Can you work these out from the model? Positions are in its coordinate system, mm. A direction names the side the tool comes from. Round coordinates to 2 decimals unless told otherwise and drop trailing zeros. Write each loop counter-clockwise with the first axis right and the second up, starting at its lowest first coordinate (ties: lowest second). Pieces come first, ordered by that corner, then holes. Notation, with made-up numbers: (82, 64) - (110, 64) arc R21 ccw to (110, 76) - close; hole circle Ø11 at (48, -11.5). An arc over 180 degrees is marked (long way). One line per item, written item: value. Start each with the question number.
(1) I'm going to push flat-ended pins straight in: pin 1 Ø1.2 at (x, z) = (1, 66) entering from -Y; pin 2 Ø1 at (x, y) = (0.5, -17) entering from +Z; pin 3 Ø1.2 at (x, z) = (2, -78) entering from +Y. Where does each tip first touch, or does it pass through?
(2) I want a section at A-A on x = 3.05. List the corners of the cut face in (y, z) for me.
(3) If I drill on L1, parallel to Y at x = 2.6, z = -17.5; L2, parallel to Z at x = 1.5, y = -25; L3, parallel to Y at x = 3.15, z = 90, over which ranges is the centre line in solid material (lowest first)? Write a range as from..to.
(4) Thinking about a two-plate mould opening in Y: for faces 1 (the face through (4, 8, 1)), 2 (the face through (2, 23.8, -19.1)), 3 (the face through (2, -23.8, 19.1)), 4 (the face through (2.03, -14.51, -31.78)), which applies, +Y half, -Y half, draft (parallel to the pull), parting line (faces both ways), or undercut?
(5) I want a section at B-B on y = -8. List the corners of the cut face in (x, z) for me, plus the area to 3 significant figures.
(6) On a 3-axis mill with a long thin cutter (end or side, diameter ignored), from which of +Z, -Z, +X, -X, +Y, -Y can I reach the whole of each face in a straight line? I mean faces 5 (the face through (2, 23.8, 19.1)), 6 (the face through (2, 10, 66)), 7 (the face through (2, -10, -66)). Say none if no direction works.
(7) I want a section at C-C on z = 62. List the corners of the cut face in (x, y) for me, plus the area to 3 significant figures.
from build123d import *

# Parameters (mm, degrees)
SKETCH1_W               = 210
SKETCH1_H               = 75
BOSS_EXTRUDE1_DEPTH     = 4
SKETCH2_R               = 1.5
CUT_EXTRUDE1_DEPTH      = 5
SKETCH3_R               = 2
CUT_EXTRUDE2_DEPTH      = 5
CUT_EXTRUDE3_DEPTH      = 5
MIRROR3_COPY_1_SKETCH_R = 2
MIRROR3_COPY_1_DEPTH    = 5
MIRROR3_COPY_2_DEPTH    = 5
SKETCH5_R               = 3
CUT_EXTRUDE4_DEPTH      = 5


with BuildPart() as part:
    # Sketch1 → Boss-Extrude1 (new body)
    with BuildSketch(Plane(origin=(0, 0, 0), x_dir=(0, 0, -1), z_dir=(1, 0, 0))):
        Rectangle(SKETCH1_W, SKETCH1_H)
    extrude(amount=BOSS_EXTRUDE1_DEPTH)

    # Sketch2 → Cut-Extrude1 (cut, through all)
    with BuildSketch(Plane(origin=(4, 0, 0), x_dir=(0, 0, -1), z_dir=(1, 0, 0))):
        with Locations((-90, 0)):
            Circle(SKETCH2_R)
    cut_extrude1 = extrude(amount=-CUT_EXTRUDE1_DEPTH, mode=Mode.SUBTRACT)

    # Sketch3 → Cut-Extrude2 (cut, through all)
    with BuildSketch(Plane(origin=(4, 0, 0), x_dir=(0, 0, -1), z_dir=(1, 0, 0))):
        with Locations((-17.5, 25)):
            Circle(SKETCH3_R)
    cut_extrude2 = extrude(amount=-CUT_EXTRUDE2_DEPTH, mode=Mode.SUBTRACT)

    # Sketch4 → Cut-Extrude3 (cut, through all)
    with BuildSketch(Plane(origin=(4, 0, 0), x_dir=(0, 0, -1), z_dir=(1, 0, 0))):
        with BuildLine():
            Line((-105, 0), (-105, 37.5))
            Line((-105, 37.5), (0, 37.5))
            Line((0, 37.5), (0, 35))
            Line((0, 35), (-17.5, 35))
            ThreePointArc((-17.5, 35), (-24.571067812, 32.071067812), (-27.5, 25))
            ThreePointArc((-27.5, 25), (-31.893398282, 14.393398282), (-42.5, 10))
            Line((-42.5, 10), (-90, 10))
            ThreePointArc((-90, 10), (-97.071067812, 7.071067812), (-100, 0))
            Line((-100, 0), (-105, 0))
        make_face()
    cut_extrude3 = extrude(amount=-CUT_EXTRUDE3_DEPTH, mode=Mode.SUBTRACT)

    # Mirror2: Cut-Extrude2, Cut-Extrude3 across plane
    add(cut_extrude2.mirror(Plane.ZX), mode=Mode.SUBTRACT)
    add(cut_extrude3.mirror(Plane.ZX), mode=Mode.SUBTRACT)

    # Mirror3: Cut-Extrude3, Cut-Extrude1, Cut-Extrude2 across plane
    add(cut_extrude3.mirror(Plane.XY), mode=Mode.SUBTRACT)
    add(cut_extrude1.mirror(Plane.XY), mode=Mode.SUBTRACT)
    add(cut_extrude2.mirror(Plane.XY), mode=Mode.SUBTRACT)

    # Mirror3 copy 1 sketch → Mirror3 copy 1 (cut, through all)
    with BuildSketch(Plane(origin=(4, 0, 0), x_dir=(0, 0, 1), z_dir=(1, 0, 0))):
        with Locations((-17.5, 25)):
            Circle(MIRROR3_COPY_1_SKETCH_R)
    extrude(amount=-MIRROR3_COPY_1_DEPTH, mode=Mode.SUBTRACT)

    # Mirror3 copy 2 sketch → Mirror3 copy 2 (cut, through all)
    with BuildSketch(Plane(origin=(4, 0, 0), x_dir=(0, 0, 1), z_dir=(1, 0, 0))):
        with BuildLine():
            Line((-105, 0), (-105, 37.5))
            Line((-105, 37.5), (0, 37.5))
            Line((0, 37.5), (0, 35))
            Line((0, 35), (-17.5, 35))
            ThreePointArc((-17.5, 35), (-24.571067812, 32.071067812), (-27.5, 25))
            ThreePointArc((-27.5, 25), (-31.893398282, 14.393398282), (-42.5, 10))
            Line((-42.5, 10), (-90, 10))
            ThreePointArc((-90, 10), (-97.071067812, 7.071067812), (-100, 0))
            Line((-100, 0), (-105, 0))
        make_face()
    extrude(amount=-MIRROR3_COPY_2_DEPTH, mode=Mode.SUBTRACT)

    # Sketch5 → Cut-Extrude4 (cut, through all)
    with BuildSketch(Plane(origin=(4, 0, 0), x_dir=(0, 0, -1), z_dir=(1, 0, 0))):
        Circle(SKETCH5_R)
    extrude(amount=-CUT_EXTRUDE4_DEPTH, mode=Mode.SUBTRACT)


solid = part.part
Established:
1. pin 1: y = -10
1. pin 2: z = 30.14
1. pin 3: y = 10
2. outline: (-35, -17.5) arc R10 ccw to (-25, -27.5) arc R15 cw to (-10, -42.5) - (-10, -90) arc R10 ccw to (10, -90) - (10, -42.5) arc R15 cw to (25, -27.5) arc R10 ccw to (35, -17.5) - (35, 17.5) arc R10 ccw to (25, 27.5) arc R15 cw to (10, 42.5) - (10, 90) arc R10 ccw to (-10, 90) - (-10, 42.5) arc R15 cw to (-25, 27.5) arc R10 ccw to (-35, 17.5) - close; hole circle Ø4 at (-25, -17.5); hole circle Ø4 at (-25, 17.5); hole circle Ø6 at (0, 0); hole circle Ø3 at (0, -90); hole circle Ø3 at (0, 90); hole circle Ø4 at (25, -17.5); hole circle Ø4 at (25, 17.5)
3. L1: -35..-27, -23..23, 27..35
3. L2: -27.5..-19.5, -15.5..15.5, 19.5..27.5
3. L3: -10..-1.5, 1.5..10
4. face 1: draft
4. face 2: undercut
4. face 3: undercut
4. face 4: -Y half
5. outline: (0, -96) - (4, -96) - (4, 96) - (0, 96) - close
5. area: 768 mm2
6. face 5: +X, -X
6. face 6: +Z, +X, -X, +Y
6. face 7: -Z, +X, -X, -Y
7. outline: (0, -10) - (4, -10) - (4, 10) - (0, 10) - close
7. area: 80.0 mm2
